```python
from build123d import *

# Parameters (mm, degrees)
SKETCH_1_W          = 43.7
SKETCH_1_H          = 11.35
EXTRUDE_1_DEPTH     = 1.7
SKETCH_2_OUTSIDE_W  = 54.736
SKETCH_2_OUTSIDE_H  = 22.386
CUT_EXTRUDE_3_DEPTH = 23.638863156
EXTRUDE_4_DEPTH     = 1.4


with BuildPart() as part:
    # Эскиз1 → Вытянуть1 (new body)
    with BuildSketch(Plane.XY):
        Rectangle(SKETCH_1_W, SKETCH_1_H)
    extrude(amount=EXTRUDE_1_DEPTH)

    # Эскиз2 outside → Вытянуть3 (cut, through all)
    with BuildSketch(Plane.XY.offset(1.7)):
        Rectangle(SKETCH_2_OUTSIDE_W, SKETCH_2_OUTSIDE_H)
        with BuildLine():
            ThreePointArc((39.456233665, 0), (0, 5.675), (-39.456233665, 0))
            ThreePointArc((-39.456233665, 0), (0, -5.675), (39.456233665, 0))
        make_face(mode=Mode.SUBTRACT)
    extrude(amount=-CUT_EXTRUDE_3_DEPTH, mode=Mode.SUBTRACT)

    # Эскиз3 → Вытянуть4 (add)
    with BuildSketch(Plane.XY.offset(1.7)):
        with BuildLine():
            Line((-9.85, 3.755003836), (9.85, 3.755003836))
            ThreePointArc((9.85, 3.755003836), (14.829805552, 3.440833038), (19.8, 3))
            Line((19.8, 3), (19.8, -3))
            ThreePointArc((19.8, -3), (14.829805552, -3.440833038), (9.85, -3.755003836))
            Line((9.85, -3.755003836), (-9.85, -3.755003836))
            ThreePointArc((-9.85, -3.755003836), (-14.829805552, -3.440833038), (-19.8, -3))
            Line((-19.8, -3), (-19.8, 3))
            ThreePointArc((-19.8, 3), (-14.829805552, 3.440833038), (-9.85, 3.755003836))
        make_face()
    extrude(amount=EXTRUDE_4_DEPTH)


solid = part.part
```
Input: part model. Units: mm. Frame: model coordinates. A direction names the side the tool comes from. Coordinates: 2 decimals unless noted, no trailing zeros. Write each loop counter-clockwise with the first axis right and the second up, starting at its lowest first coordinate (ties: lowest second). Pieces come first, ordered by that corner, then holes. Notation, with made-up numbers: (-17, 69) -> (10, 69) arc R21 cw to (10, 96) -> close; hole circle Ø1 at (77, 55.25). An arc over 180 degrees is marked (long way). Write each question's results on one line, items separated by ' | '.
Item 1: Section query B-B on z = 2.2. Return loops of the section in (x, y) (3 decimals), plus the area to 3 significant figures.
Conclusion:
outline: (-19.8, -3) arc R196 ccw to (-9.85, -3.755) -> (9.85, -3.755) arc R196 ccw to (19.8, -3) -> (19.8, 3) arc R196 ccw to (9.85, 3.755) -> (-9.85, 3.755) arc R196 ccw to (-19.8, 3) -> close | area: 284 mm^2
Item 2: Section query A-A on y = 0. Return loops of the section in (x, z).
Conclusion:
outline: (-21.85, 0) -> (21.85, 0) -> (21.85, 1.7) -> (19.8, 1.7) -> (19.8, 3.1) -> (-19.8, 3.1) -> (-19.8, 1.7) -> (-21.85, 1.7) -> close
Item 3: Pin query (flat end, axial travel): pin 1 Ø1.5 at (y, z) = (0, 3) entering from -X; pin 2 Ø1.1 at (y, z) = (0, 2.5) entering from +X. Return the tip coordinate at first contact, or that it passes through.
Conclusion:
pin 1: stops at x = -19.8 | pin 2: stops at x = 19.8
Item 4: Section query C-C on y = 4.5. Return loops of the section in (x, z).
Conclusion:
outline: (-18.1, 0) -> (18.1, 0) -> (18.1, 1.7) -> (-18.1, 1.7) -> close
Item 5: Material intervals for probe 1 along X at (y, z) = (1.75, 2.4); probe 2 along Z at (x, y) = (-6, -4); probe 3 along Y at (x, z) = (6.5, 2.8) (3 decimals), sorted ascending.
Conclusion:
probe 1: x = -19.8 to 19.8 | probe 2: z = 0 to 1.7 | probe 3: y = -3.755 to 3.755
Item 6: Set-up query: faces 1 (the cylindrical face through (14.899, -3.436, 2.39)), 2 (the flat face through (0, -3.755, 2)), 3 (the flat face through (-19.8, 0, 2)), 4 (the cylindrical face through (14.76, 3.446, 2.39)). Return all of +Z, -Z, +X, -X, +Y, -Y with unobstructed straight access to the full face (end or side cutting, diameter ignored); none if empty.
Conclusion:
face 1: +Z, +X, -Y | face 2: +Z, +X, -X, -Y | face 3: +Z, -X, +Y, -Y | face 4: +Z, +X, +Y
